from build123d import *

# Parameters (mm, degrees)
F0_W     = 203.2
F0_H     = 127
F1_DEPTH = 127
F3_DEPTH = 76.2
F4_SIZE2 = 101.6
F4_SIZE  = 76.2
F5_R     = 5.08
F6_R     = 15.24
F7_DEPTH = 50.8
F8_R     = 14.4150748184
F9_DEPTH = 127


with BuildPart() as f1:
    # F0 (on Front) → F1 (new body)
    with BuildSketch(Plane.XZ):
        with Locations((-6.4546563804, 2.2225044668)):
            Rectangle(F0_W, F0_H)
    extrude(amount=F1_DEPTH)

    # F2 (on face) → F3 (cut)
    with BuildSketch(Plane.XZ.offset(127)):
        Polygon((95.1453436196, 65.7225044668), (-6.4546563804, 65.7225044668), (-6.4546563804, 0), (-44.5546563804, 0), (-44.5546563804, -61.2774955332), (95.1453436196, -61.2774955332), align=None)
    extrude(amount=-F3_DEPTH, mode=Mode.SUBTRACT)

    # F4
    f4_edges = [f1.edges().sort_by_distance(p)[0] for p in [
        (95.145344, -25.4, 65.722504),
    ]]
    f4_side = f1.faces().sort_by_distance((-28.226085, -52.614286, 65.722504))[0]
    chamfer(f4_edges, length=F4_SIZE, length2=F4_SIZE2, reference=f4_side)

    # F5
    f5_edges = [f1.edges().sort_by_distance(p)[0] for p in [
        (-6.454656, -88.9, 65.722504),
        (-57.254656, -127, 65.722504),
        (-6.454656, -127, 32.861252),
        (-6.454656, -88.9, 0),
        (-6.454656, -50.8, 32.861252),
        (18.945344, -25.4, 65.722504),
        (-44.554656, 0, 65.722504),
        (-108.054656, -63.5, 65.722504),
        (6.245344, -50.8, 65.722504),
        (-25.504656, -127, 0),
        (-44.554656, -127, -30.638748),
        (-76.304656, -127, -61.277496),
        (-108.054656, -127, 2.222504),
        (-44.554656, -88.9, 0),
        (-44.554656, -88.9, -61.277496),
        (-44.554656, -50.8, -30.638748),
        (-6.454656, 0, -61.277496),
        (95.145344, -25.4, -61.277496),
        (25.295344, -50.8, -61.277496),
        (-108.054656, -63.5, -61.277496),
        (-108.054656, 0, 2.222504),
        (-25.504656, -50.8, 0),
    ]]
    fillet(f5_edges, radius=F5_R)

    # F6 (on face) → F7 (cut, through all)
    with BuildSketch(Plane.XZ.offset(50.8)):
        with Locations((11.3253436196, -15.5574955332)):
            Circle(F6_R)
    extrude(amount=-F7_DEPTH, mode=Mode.SUBTRACT)

    # F8 (on face) → F9 (cut, through all)
    with BuildSketch(Plane.XY.offset(65.7225044668)):
        with Locations((-76.158054173, -93.8184931874)):
            Circle(F8_R)
    extrude(amount=-F9_DEPTH, mode=Mode.SUBTRACT)


solid = f1.part
Part model, mm, in its own coordinate system. A direction names the side the tool comes from. Round coordinates to 2 decimals unless told otherwise and drop trailing zeros. Order: outer loops, then holes, each group sorted by start corner. A loop starts at its lowest first (then second) coordinate and runs counter-clockwise, first axis right, second up. Notation, with made-up numbers: (-22, 72) -> (2, 72) arc R26 ccw to (2, 102) -> close; hole circle Ø8 at (66.25, 44). An arc over 180 degrees is marked (long way). Put each result on its own line as item: value.
Q1. Wall check: line 1 (X direction, y = -119.5, z = -42); line 2 (Y direction, x = 15.5, z = -54.5); line 3 (Z direction, x = -19.5, y = -57). Give the ranges that are in metal, low to high. Write a range as [from, to].
From the geometry:
line 1: x = [-108.05, -44.55]
line 2: y = [-50.8, 0]
line 3: z = [0, 65.72]
Q2. Band-saw the part on B-B (y = -91). Give the cut face in (x, z).
From the geometry:
outline: (-108.05, -56.2) arc R5.08 ccw to (-102.97, -61.28) -> (-90.29, -61.28) -> (-90.29, 65.72) -> (-102.97, 65.72) arc R5.08 ccw to (-108.05, 60.64) -> close; (-62.02, -61.28) -> (-49.63, -61.28) arc R5.08 ccw to (-44.55, -56.2) -> (-44.55, -5.08) arc R5.08 cw to (-39.47, 0) -> (-11.53, 0) arc R5.08 ccw to (-6.45, 5.08) -> (-6.45, 60.64) arc R5.08 ccw to (-11.53, 65.72) -> (-62.02, 65.72) -> close
Q3. Band-saw the part on C-C (z = -10). Give the cut face in (x, y), and give its area (3 significant figures).
From the geometry:
outline: (-108.05, -121.92) arc R5.08 ccw to (-102.97, -127) -> (-49.63, -127) arc R5.08 ccw to (-44.55, -121.92) -> (-44.55, -55.88) arc R5.08 cw to (-39.47, -50.8) -> (-2.87, -50.8) -> (-2.87, 0) -> (-102.97, 0) arc R5.08 ccw to (-108.05, -5.08) -> close; (25.52, -50.8) -> (75.74, -50.8) -> (75.74, 0) -> (25.52, 0) -> close; hole circle Ø28.83 at (-76.16, -93.82)
area: 12,100 mm2
Q4. Tool access for faces 1 (the face through (-43.03, -88.44, -1.45)), 2 (the face through (-68.409, -81.664, 3.112)): list every direction of +Z, -Z, +X, -X, +Y, -Y with a clear straight run to the whole face (end or side of a thin tool).
From the geometry:
face 1: -Z, +X, -Y
face 2: +Z, -Z
Q5. Band-saw the part on D-D (x = -87). Give the cut face in (y, z).
From the geometry:
outline: (-127, -56.2) arc R5.08 ccw to (-121.92, -61.28) -> (-103.32, -61.28) -> (-103.32, 65.72) -> (-121.92, 65.72) arc R5.08 ccw to (-127, 60.64) -> close; (-84.32, -61.28) -> (-5.08, -61.28) arc R5.08 ccw to (0, -56.2) -> (0, 60.64) arc R5.08 ccw to (-5.08, 65.72) -> (-84.32, 65.72) -> close
Q6. Pin check, flat tips, straight feed: pin 1 Ø8.5 at (x, y) = (-28, -81) entering from -Z; pin 2 Ø16.5 at (y, z) = (-73, 21.5) entering from +X; pin 3 Ø2 at (x, z) = (21.5, -8.5) entering from +Y (1 decimal); pin 4 Ø4 at (x, z) = (44.5, -36) entering from -Y. Stop position of each tip, or through.
From the geometry:
pin 1: stops at z = 0
pin 2: stops at x = -6.45
pin 3: passes through
pin 4: stops at y = -50.8
Q7. Band-saw the part on A-A (x = -30.5). Give the cut face in (y, z), and give its area (3 significant figures).
From the geometry:
outline: (-127, 5.08) arc R5.08 ccw to (-121.92, 0) -> (-55.88, 0) arc R5.08 cw to (-50.8, -5.08) -> (-50.8, -56.2) arc R5.08 ccw to (-45.72, -61.28) -> (-5.08, -61.28) arc R5.08 ccw to (0, -56.2) -> (0, 60.64) arc R5.08 ccw to (-5.08, 65.72) -> (-121.92, 65.72) arc R5.08 ccw to (-127, 60.64) -> close
area: 11,400 mm2
